```python
from build123d import *

# Parameters (mm, degrees)
SKETCH1_W                       = 145
SKETCH1_H                       = 106
BOSS_EXTRUDE1_DEPTH             = 16
CUT_EXTRUDE1_START              = 16
SKETCH1_4_W                     = 125
SKETCH1_4_H                     = 86
CUT_EXTRUDE1_DEPTH              = 6
SKETCH6_W                       = 10
SKETCH6_H                       = 10
BOSS_EXTRUDE5_DEPTH             = 3
MIRROR2_COPY_1_SKETCH_W         = 10
MIRROR2_COPY_1_SKETCH_H         = 10
MIRROR2_COPY_1_DEPTH            = 3
BOSS_EXTRUDE6_REACH             = 93.221
BOSS_EXTRUDE6_DIRECTION_2_REACH = 93.221
BOSS_EXTRUDE7_REACH             = 94.229
SKETCH9_W                       = 5
SKETCH9_H                       = 11
BOSS_EXTRUDE7_DIRECTION_2_REACH = 94.229
FILLET1_R                       = 10
FILLET3_R                       = 2
FILLET11_R                      = 1


with BuildPart() as part:
    # Sketch1 → Boss-Extrude1 (new body)
    with BuildSketch(Plane(origin=(0, 0, 0), x_dir=(1, 0, 0), z_dir=(0, 1, 0))):
        Rectangle(SKETCH1_W, SKETCH1_H)
    extrude(amount=BOSS_EXTRUDE1_DEPTH)

    # Sketch1<4> → Cut-Extrude1 (cut)
    with BuildSketch(Plane(origin=(0, 0, 0), x_dir=(1, 0, 0), z_dir=(0, 1, 0)).offset(CUT_EXTRUDE1_START)):
        Rectangle(SKETCH1_4_W, SKETCH1_4_H)
    extrude(amount=-CUT_EXTRUDE1_DEPTH, mode=Mode.SUBTRACT)

    # Sketch6 → Boss-Extrude5 (add)
    with BuildSketch(Plane(origin=(0, 10, 0), x_dir=(1, 0, 0), z_dir=(0, 1, 0))):
        with Locations((-57.5, 38)):
            Rectangle(SKETCH6_W, SKETCH6_H)
    boss_extrude5 = extrude(amount=BOSS_EXTRUDE5_DEPTH)

    # Sketch8 → M4 Clearance Hole1 (revolve, cut)
    with BuildSketch(Plane(origin=(-57.5, 13, -38), x_dir=(0, 0, 1), z_dir=(1, 0, 0))):
        Polygon((0, 0), (0, 7.25), (2.25, 5), (2.25, 0), align=None)
    m4_clearance_hole1 = revolve(axis=Axis((-57.5, 19.35, -38), (0, -1, 0)), mode=Mode.SUBTRACT)

    # Mirror1: Boss-Extrude5, M4 Clearance Hole1 across plane
    add(boss_extrude5.mirror(Plane(origin=(0, 0, 0), x_dir=(0, 0, 1), z_dir=(1, 0, 0))))
    add(m4_clearance_hole1.mirror(Plane(origin=(0, 0, 0), x_dir=(0, 0, 1), z_dir=(1, 0, 0))), mode=Mode.SUBTRACT)

    # Mirror2: Boss-Extrude5, M4 Clearance Hole1 across plane
    add(boss_extrude5.mirror(Plane.XY))
    add(m4_clearance_hole1.mirror(Plane.XY), mode=Mode.SUBTRACT)

    # Mirror2 copy 1 sketch → Mirror2 copy 1 (add)
    with BuildSketch(Plane(origin=(0, 10, 0), x_dir=(-1, 0, 0), z_dir=(0, 1, 0))):
        with Locations((-57.5, 38)):
            Rectangle(MIRROR2_COPY_1_SKETCH_W, MIRROR2_COPY_1_SKETCH_H)
    extrude(amount=MIRROR2_COPY_1_DEPTH)

    # Mirror2 copy 2 sketch → Mirror2 copy 2 (revolve, cut)
    with BuildSketch(Plane(origin=(57.5, 13, 38), x_dir=(0, 0, -1), z_dir=(-1, 0, 0))):
        Polygon((0, 0), (0, 7.25), (2.25, 5), (2.25, 0), align=None)
    revolve(axis=Axis((57.5, 19.35, 38), (0, -1, 0)), mode=Mode.SUBTRACT)

    # Boss-Extrude6: up to this face of the body (flat: up to its plane)
    boss_extrude6_end = Plane(part.part.faces().sort_by_distance((-57.5, 11.5, -33))[0])
    # Sketch4 → Boss-Extrude6 (add, up to the picked face)
    with BuildSketch(Plane.XY, mode=Mode.PRIVATE) as boss_extrude6_sk1:
        Polygon((-57.5, 10), (-57.5, 21), (-62.5, 21), (-62.5, 16), (-62.5, 10), align=None)
    boss_extrude6_tool1 = split(extrude(boss_extrude6_sk1.sketch, amount=-BOSS_EXTRUDE6_REACH, mode=Mode.PRIVATE), bisect_by=boss_extrude6_end, keep=Keep.BOTH, mode=Mode.PRIVATE)
    boss_extrude6 = boss_extrude6_tool1.solids().sort_by(Axis((-60, 15.5, 0), (0, 0, -1)))[0]
    add(boss_extrude6)

    # Boss-Extrude6 direction 2: up to this face of the body (flat: up to its plane)
    boss_extrude6_direction_2_end = Plane(part.part.faces().sort_by_distance((-57.5, 11.5, 33))[0])
    # Sketch4 → Boss-Extrude6 direction 2 (add, up to the picked face)
    with BuildSketch(Plane.XY, mode=Mode.PRIVATE) as boss_extrude6_direction_2_sk1:
        Polygon((-57.5, 10), (-57.5, 21), (-62.5, 21), (-62.5, 16), (-62.5, 10), align=None)
    boss_extrude6_direction_2_tool1 = split(extrude(boss_extrude6_direction_2_sk1.sketch, amount=BOSS_EXTRUDE6_DIRECTION_2_REACH, mode=Mode.PRIVATE), bisect_by=boss_extrude6_direction_2_end, keep=Keep.BOTH, mode=Mode.PRIVATE)
    boss_extrude6_direction_2 = boss_extrude6_direction_2_tool1.solids().sort_by(Axis((-60, 15.5, 0), (0, 0, 1)))[0]
    add(boss_extrude6_direction_2)

    # Boss-Extrude7: up to this face of the body (flat: up to its plane)
    boss_extrude7_end = Plane(part.part.faces().sort_by_distance((52.5, 11.5, 38))[0])
    # Sketch9 → Boss-Extrude7 (add, up to the picked face)
    with BuildSketch(Plane(origin=(0, 0, 0), x_dir=(0, 0, -1), z_dir=(1, 0, 0)), mode=Mode.PRIVATE) as boss_extrude7_sk1:
        with Locations((-40.5, 15.5)):
            Rectangle(SKETCH9_W, SKETCH9_H)
    boss_extrude7_tool1 = split(extrude(boss_extrude7_sk1.sketch, amount=BOSS_EXTRUDE7_REACH, mode=Mode.PRIVATE), bisect_by=boss_extrude7_end, keep=Keep.BOTH, mode=Mode.PRIVATE)
    boss_extrude7 = boss_extrude7_tool1.solids().sort_by(Axis((0, 15.5, 40.5), (1, 0, 0)))[0]
    add(boss_extrude7)

    # Boss-Extrude7 direction 2: up to this face of the body (flat: up to its plane)
    boss_extrude7_direction_2_end = Plane(part.part.faces().sort_by_distance((-52.5, 11.5, 38))[0])
    # Sketch9 → Boss-Extrude7 direction 2 (add, up to the picked face)
    with BuildSketch(Plane(origin=(0, 0, 0), x_dir=(0, 0, -1), z_dir=(1, 0, 0)), mode=Mode.PRIVATE) as boss_extrude7_direction_2_sk1:
        with Locations((-40.5, 15.5)):
            Rectangle(SKETCH9_W, SKETCH9_H)
    boss_extrude7_direction_2_tool1 = split(extrude(boss_extrude7_direction_2_sk1.sketch, amount=-BOSS_EXTRUDE7_DIRECTION_2_REACH, mode=Mode.PRIVATE), bisect_by=boss_extrude7_direction_2_end, keep=Keep.BOTH, mode=Mode.PRIVATE)
    boss_extrude7_direction_2 = boss_extrude7_direction_2_tool1.solids().sort_by(Axis((0, 15.5, 40.5), (-1, 0, 0)))[0]
    add(boss_extrude7_direction_2)

    # Mirror3: Boss-Extrude6, Boss-Extrude6 direction 2 across plane
    add(boss_extrude6.mirror(Plane(origin=(0, 0, 0), x_dir=(0, 0, 1), z_dir=(1, 0, 0))))
    add(boss_extrude6_direction_2.mirror(Plane(origin=(0, 0, 0), x_dir=(0, 0, 1), z_dir=(1, 0, 0))))

    # Mirror4: Boss-Extrude7, Boss-Extrude7 direction 2 across plane
    add(boss_extrude7.mirror(Plane.XY))
    add(boss_extrude7_direction_2.mirror(Plane.XY))

    # Fillet1
    fillet1_edges = [part.edges().sort_by_distance(p)[0] for p in [
        (0, 0, -53),
        (72.5, 0, 0),
        (0, 0, 53),
        (-72.5, 0, 0),
        (-72.5, 8, -53),
        (72.5, 8, -53),
        (72.5, 8, 53),
        (-72.5, 8, 53),
    ]]
    fillet(fillet1_edges, radius=FILLET1_R)

    # Fillet3
    fillet3_edges = [part.edges().sort_by_distance(p)[0] for p in [
        (-55, 10, 33),
        (-55, 10, -33),
        (-57.5, 10, 0),
        (0, 10, 38),
        (55, 10, 33),
        (55, 10, -33),
        (57.5, 10, 0),
        (0, 10, -38),
        (-52.5, 10, -35.5),
        (52.5, 10, -35.5),
        (52.5, 10, 35.5),
        (-52.5, 10, 35.5),
    ]]
    fillet(fillet3_edges, radius=FILLET3_R)

    # Fillet11
    fillet11_edges = [part.edges().sort_by_distance(p)[0] for p in [
        (0, 16, 53),
        (72.5, 16, 0),
        (0, 16, -53),
        (-72.5, 16, 0),
        (-69.571067812, 16, 50.071067812),
        (69.571067812, 16, 50.071067812),
        (69.571067812, 16, -50.071067812),
        (-69.571067812, 16, -50.071067812),
    ]]
    fillet(fillet11_edges, radius=FILLET11_R)


solid = part.part
```
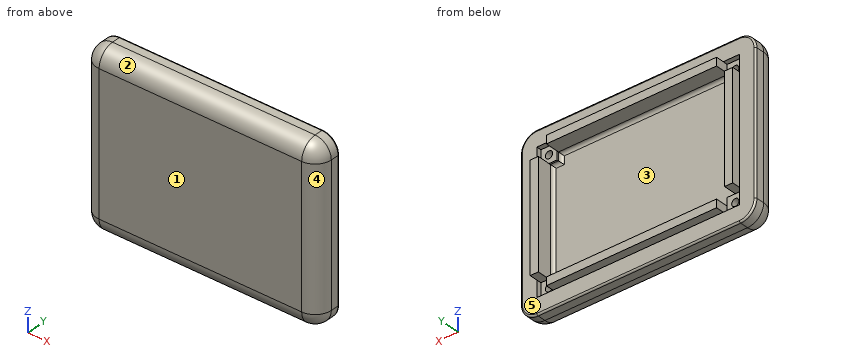
CAD build for the part. Positions are in the model's coordinates, mm. Face numbers are marked on the shaded views. A direction names the side the tool comes from. Round coordinates to 2 decimals unless told otherwise and drop trailing zeros. Loops run counter-clockwise (first coordinate to the right, second up) from the corner with the lowest first, then second, coordinate; pieces in that order, holes last. Notation, with made-up numbers: M -37.75,-19.75 L 1.25,-19.75 A28 cw 1.25,8.25 Z; hole C -24,54.25 d1. An arc over 180 degrees is marked long. Use a Markdown table: item, result. Add a question column.
(1) Cut at B-B (z = -9). Give the cut face in (x, y).
(2) Which spindle directions (+Z, -Z, +X, -X, +Y, -Y) get a long thin tool onto all of the face, cutting with end or side? Do the marked faces 4 and 5. Say none if no direction does.
(3) Cut at C-C (x = 44). Give the cut face in (y, z).
(4) Cut at A-A (y = 17.75). Give the cut face in (x, z).
(5) Cut at D-D (y = 3.25). Give the cut face in (x, z).
(6) Flat gauge pins, fed straight in: pin 1 (7 mm diameter, centred on y = 17.5, z = 1.5, fed in from -X); pin 2 (1.5 mm diameter, centred on y = 18.5, z = -40.5, fed in from +X); pin 3 (2.5 mm diameter, centred on x = 1, y = 17.5, fed in from -Z); pin 4 (1.5 mm diameter, centred on x = -61, y = 19, fed in from -Z). Where does each tip first touch, or does it go through?
(7) Pull direction Z, two halves, no side cores. Call the marked faces 1, 2 and 3: +Z half, -Z half, draft (parallel to the pull), parting line (faces both ways), or undercut.
(8) Drill centre lines: line 1 (Z direction, x = -57.5, y = 10.9); line 2 (Z direction, x = 17, y = 19.5); line 3 (X direction, y = 13.5, z = 20.5). Where is each one in solid material? Low to high.
Geometry says:
| question | item | result |
|---|---|---|
| 1 | outline | M -72.5,10 A10 ccw -62.5,0 L 62.5,0 A10 ccw 72.5,10 L 72.5,15 A1 ccw 71.5,16 L 62.5,16 L 62.5,21 L 57.5,21 L 57.5,12 A2 cw 55.5,10 L -55.5,10 A2 cw -57.5,12 L -57.5,21 L -62.5,21 L -62.5,16 L -71.5,16 A1 ccw -72.5,15 Z |
| 2 | face 4 | +Z, -Z, +X, -Y |
| 2 | face 5 | +Y |
| 3 | outline | M 0,-43 A10 ccw 10,-53 L 15,-53 A1 ccw 16,-52 L 16,-43 L 21,-43 L 21,-38 L 12,-38 A2 cw 10,-36 L 10,36 A2 cw 12,38 L 21,38 L 21,43 L 16,43 L 16,52 A1 ccw 15,53 L 10,53 A10 ccw 0,43 Z |
| 4 | outline | M -62.5,-33 L -57.5,-33 L -57.5,33 L -62.5,33 Z; M -52.5,-43 L 52.5,-43 L 52.5,-38 L -52.5,-38 Z; M -52.5,38 L 52.5,38 L 52.5,43 L -52.5,43 Z; M 57.5,-33 L 62.5,-33 L 62.5,33 L 57.5,33 Z |
| 5 | outline | M -69.88,-43 A7.38 ccw -62.5,-50.38 L 62.5,-50.38 A7.38 ccw 69.88,-43 L 69.88,43 A7.38 ccw 62.5,50.38 L -62.5,50.38 A7.38 ccw -69.88,43 Z |
| 6 | pin 1 | stops at x = -72.5 |
| 6 | pin 2 | stops at x = 52.5 |
| 6 | pin 3 | stops at z = -43 |
| 6 | pin 4 | stops at z = -33 |
| 7 | face 1 | draft |
| 7 | face 2 | +Z half |
| 7 | face 3 | undercut |
| 8 | line 1 | z = -53 to -40.25, -35.75 to 35.75, 40.25 to 53 |
| 8 | line 2 | z = -43 to -38, 38 to 43 |
| 8 | line 3 | x = -72.5 to -57.5, 57.5 to 72.5 |
